Geometry check sheet. Reference: the model listing, model coordinates, mm. Give positions to 0.01 mm unless a question says otherwise; leave off trailing zeros. Loops run counter-clockwise (first coordinate to the right, second up) from the corner with the lowest first, then second, coordinate; pieces in that order, holes last. Notation, with made-up numbers: (71, -4) -> (130, -4) arc R27 ccw to (130, 22) -> close; hole circle Ø3 at (60, 46). An arc over 180 degrees is marked (long way). Write item = value, one per line.
```python
from build123d import *

# Parameters (mm, degrees)
BOSS_EXTRUDE1_DEPTH = 10
CUT_EXTRUDE1_REACH  = 34.319
SKETCH4_R           = 5.25
CUT_EXTRUDE2_REACH  = 34.319
SKETCH6_R           = 1.75
CUT_EXTRUDE3_REACH  = 34.319
SKETCH7_R           = 1.75
FILLET1_R           = 2


with BuildPart() as part:
    # Sketch2 → Boss-Extrude1 (new body)
    with BuildSketch(Plane.XY):
        with BuildLine():
            Line((11.5, -17), (-11.5, -17))
            Line((-11.5, -17), (-11.5, 17))
            ThreePointArc((-11.5, 17), (0, 28.5), (11.5, 17))
            Line((11.5, 17), (11.5, -17))
        make_face()
    extrude(amount=BOSS_EXTRUDE1_DEPTH)

    # Sketch4 → Cut-Extrude1 (cut, up to next)
    with BuildSketch(Plane.XY.offset(10), mode=Mode.PRIVATE) as cut_extrude1_sk1:
        with Locations((0, 17)):
            Circle(SKETCH4_R)
    cut_extrude1_tool1 = extrude(cut_extrude1_sk1.sketch, amount=-CUT_EXTRUDE1_REACH, mode=Mode.PRIVATE) & part.part
    add(cut_extrude1_tool1.solids().sort_by_distance((0, 17, 10))[0], mode=Mode.SUBTRACT)

    # Sketch6 → Cut-Extrude2 (cut, up to next)
    with BuildSketch(Plane(origin=(0, 0, 0), x_dir=(-1, 0, 0), z_dir=(0, 0, -1)), mode=Mode.PRIVATE) as cut_extrude2_sk1:
        with Locations((0, 25)):
            Circle(SKETCH6_R)
    cut_extrude2_tool1 = extrude(cut_extrude2_sk1.sketch, amount=-CUT_EXTRUDE2_REACH, mode=Mode.PRIVATE) & part.part
    # Sketch6 → Cut-Extrude2 (cut, up to next)
    with BuildSketch(Plane(origin=(0, 0, 0), x_dir=(-1, 0, 0), z_dir=(0, 0, -1)), mode=Mode.PRIVATE) as cut_extrude2_sk2:
        with Locations((8, 17)):
            Circle(SKETCH6_R)
    cut_extrude2_tool2 = extrude(cut_extrude2_sk2.sketch, amount=-CUT_EXTRUDE2_REACH, mode=Mode.PRIVATE) & part.part
    # Sketch6 → Cut-Extrude2 (cut, up to next)
    with BuildSketch(Plane(origin=(0, 0, 0), x_dir=(-1, 0, 0), z_dir=(0, 0, -1)), mode=Mode.PRIVATE) as cut_extrude2_sk3:
        with Locations((0, 9)):
            Circle(SKETCH6_R)
    cut_extrude2_tool3 = extrude(cut_extrude2_sk3.sketch, amount=-CUT_EXTRUDE2_REACH, mode=Mode.PRIVATE) & part.part
    # Sketch6 → Cut-Extrude2 (cut, up to next)
    with BuildSketch(Plane(origin=(0, 0, 0), x_dir=(-1, 0, 0), z_dir=(0, 0, -1)), mode=Mode.PRIVATE) as cut_extrude2_sk4:
        with Locations((-8, 17)):
            Circle(SKETCH6_R)
    cut_extrude2_tool4 = extrude(cut_extrude2_sk4.sketch, amount=-CUT_EXTRUDE2_REACH, mode=Mode.PRIVATE) & part.part
    add(cut_extrude2_tool1.solids().sort_by_distance((0, 25, 0))[0], mode=Mode.SUBTRACT)
    add(cut_extrude2_tool2.solids().sort_by_distance((-8, 17, 0))[0], mode=Mode.SUBTRACT)
    add(cut_extrude2_tool3.solids().sort_by_distance((0, 9, 0))[0], mode=Mode.SUBTRACT)
    add(cut_extrude2_tool4.solids().sort_by_distance((8, 17, 0))[0], mode=Mode.SUBTRACT)

    # Sketch7 → Cut-Extrude3 (cut, up to next)
    with BuildSketch(Plane(origin=(0, 0, 0), x_dir=(-1, 0, 0), z_dir=(0, 0, -1)), mode=Mode.PRIVATE) as cut_extrude3_sk1:
        with Locations((-6.5, -3)):
            Circle(SKETCH7_R)
    cut_extrude3_tool1 = extrude(cut_extrude3_sk1.sketch, amount=-CUT_EXTRUDE3_REACH, mode=Mode.PRIVATE) & part.part
    # Sketch7 → Cut-Extrude3 (cut, up to next)
    with BuildSketch(Plane(origin=(0, 0, 0), x_dir=(-1, 0, 0), z_dir=(0, 0, -1)), mode=Mode.PRIVATE) as cut_extrude3_sk2:
        with Locations((6.5, -3)):
            Circle(SKETCH7_R)
    cut_extrude3_tool2 = extrude(cut_extrude3_sk2.sketch, amount=-CUT_EXTRUDE3_REACH, mode=Mode.PRIVATE) & part.part
    # Sketch7 → Cut-Extrude3 (cut, up to next)
    with BuildSketch(Plane(origin=(0, 0, 0), x_dir=(-1, 0, 0), z_dir=(0, 0, -1)), mode=Mode.PRIVATE) as cut_extrude3_sk3:
        with Locations((6.5, -13)):
            Circle(SKETCH7_R)
    cut_extrude3_tool3 = extrude(cut_extrude3_sk3.sketch, amount=-CUT_EXTRUDE3_REACH, mode=Mode.PRIVATE) & part.part
    # Sketch7 → Cut-Extrude3 (cut, up to next)
    with BuildSketch(Plane(origin=(0, 0, 0), x_dir=(-1, 0, 0), z_dir=(0, 0, -1)), mode=Mode.PRIVATE) as cut_extrude3_sk4:
        with Locations((-6.5, -13)):
            Circle(SKETCH7_R)
    cut_extrude3_tool4 = extrude(cut_extrude3_sk4.sketch, amount=-CUT_EXTRUDE3_REACH, mode=Mode.PRIVATE) & part.part
    add(cut_extrude3_tool1.solids().sort_by_distance((6.5, -3, 0))[0], mode=Mode.SUBTRACT)
    add(cut_extrude3_tool2.solids().sort_by_distance((-6.5, -3, 0))[0], mode=Mode.SUBTRACT)
    add(cut_extrude3_tool3.solids().sort_by_distance((-6.5, -13, 0))[0], mode=Mode.SUBTRACT)
    add(cut_extrude3_tool4.solids().sort_by_distance((6.5, -13, 0))[0], mode=Mode.SUBTRACT)

    # Fillet1
    fillet1_edges = [part.edges().sort_by_distance(p)[0] for p in [
        (11.5, -17, 5),
        (-11.5, -17, 5),
    ]]
    fillet(fillet1_edges, radius=FILLET1_R)


solid = part.part
```
Item 1: Draft check along X on faces 1 (the cylindrical face through (-7.772, 18.735, 4.93)), 2 (the flat face through (-11.5, 1, 5)), 3 (the flat face through (0, 6, 0)). Enter one of: +X half, -X half, draft (parallel to the pull), parting line (faces both ways), or undercut.
Answer:
face_1 = undercut
face_2 = -X half
face_3 = draft
Item 2: Section check D-D, the plane y = 25. Record the cut outline in (x, z), plus the area to 3 significant figures.
Answer:
outline = (-8.26, 0) -> (-1.75, 0) -> (-1.75, 10) -> (-8.26, 10) -> close; (1.75, 0) -> (8.26, 0) -> (8.26, 10) -> (1.75, 10) -> close
area = 130 mm^2
Item 3: Gauge pin test, flat ends, axial feed: pin 1 (13.5 mm diameter, centred on x = 0, y = 17, fed in from +Z); pin 2 (6 mm diameter, centred on x = -1.5, y = 16.5, fed in from -Z); pin 3 (1 mm diameter, centred on x = 8.5, z = 8, fed in from +Y). Record the tip position at first contact, or that the pin passes through.
Answer:
pin_1 = 10
pin_2 = through
pin_3 = 25.26
Item 4: Section check B-B, the plane x = 0. Record the cut outline in (y, z).
Answer:
outline = (-17, 0) -> (7.25, 0) -> (7.25, 10) -> (-17, 10) -> close; (10.75, 0) -> (11.75, 0) -> (11.75, 10) -> (10.75, 10) -> close; (22.25, 0) -> (23.25, 0) -> (23.25, 10) -> (22.25, 10) -> close; (26.75, 0) -> (28.5, 0) -> (28.5, 10) -> (26.75, 10) -> close
Item 5: Section check A-A, the plane y = -3. Record the cut outline in (x, z), plus the area to 3 significant figures.
Answer:
outline = (-11.5, 0) -> (-8.25, 0) -> (-8.25, 10) -> (-11.5, 10) -> close; (-4.75, 0) -> (4.75, 0) -> (4.75, 10) -> (-4.75, 10) -> close; (8.25, 0) -> (11.5, 0) -> (11.5, 10) -> (8.25, 10) -> close
area = 160 mm^2
Item 6: Thickness scan on L1, parallel to Y at x = 0, z = 2.5; L2, parallel to Y at x = -6.5, z = 5.5; L3, parallel to X at y = 13, z = 7.75. Record the ranges inside material, lowest first. Write a range as [from, to].
Answer:
L1 = [-17, 7.25], [10.75, 11.75], [22.25, 23.25], [26.75, 28.5]
L2 = [-17, -14.75], [-11.25, -4.75], [-1.25, 16.1], [17.9, 26.49]
L3 = [-11.5, -3.4], [3.4, 11.5]
Item 7: Section check C-C, the plane z = 1.75. Give the number of separate pieces and of enclosed holes in the cut face, plus the area to 3 significant figures.
Answer:
separate_pieces = 1
enclosed_holes = 9
area = 824 mm^2
